from build123d import *

# Parameters (mm, degrees)
F0_R        = 19.05
F1_DEPTH    = 44.45
F2_W        = 88.9
F2_H        = 12.7
F3_DEPTH    = 44.45
F4_T1_DEPTH = 44.45
F5_R        = 9.525
F6_DEPTH    = 44.45
F7_W        = 50.8
F7_H        = 15.3564938247
F8_DEPTH    = 12.7
F9_R        = 7.62
F10_R       = 7.62
F11_R       = 9.525
F12_R       = 9.525


# Not quite as in the source:
# - a fillet or chamfer that OpenCascade refuses, or shapes differently, is made with other operations: its cross-section is extruded or revolved along the edge and cut away or added


with BuildPart() as f1:
    # F0 (on Front) → F1 (new body)
    with BuildSketch(Plane.XZ):
        with Locations((-59.2879876494, 38.2781662047)):
            Circle(F0_R)
    extrude(amount=F1_DEPTH)

    # F2 (on Front) → F3 (join)
    with BuildSketch(Plane.XZ):
        with Locations((-15.6031847, 49.8112538493)):
            Rectangle(F2_W, F2_H)
    extrude(amount=F3_DEPTH)

    # F4: fillet of radius 6.35 on 1 edges, made by hand

    # F4_s2 → F4_t1 (join)
    with BuildSketch(Plane.XZ):
        with BuildLine():
            add(Edge.make_bspline(
                [(-40.2581018773, 37.4029819382), (-39.9794820095, 43.4612538493), (-33.91480662, 43.4612538493)],
                knots=[0, 0, 0, 1, 1, 1], degree=2, weights=[1, 1, 1]))
            Line((-33.91480662, 43.4612538493), (-40.9566455691, 43.4612538493))
            ThreePointArc((-40.9566455691, 43.4612538493), (-40.3633740127, 40.4602520649), (-40.2581018773, 37.4029819382))
        make_face()
    extrude(amount=F4_T1_DEPTH)

    # F5 (on face) → F6 (cut)
    with BuildSketch(Plane.XZ.offset(44.45)):
        with Locations((-59.2879876494, 38.2781662047)):
            Circle(F5_R)
    extrude(amount=-F6_DEPTH, mode=Mode.SUBTRACT)

    # F7 (on face) → F8 (cut)
    with BuildSketch(Plane(origin=(0, 0, 43.4612538493), x_dir=(1, 0, 0), z_dir=(0, 0, -1))):
        with Locations((3.4468153, 21.9657469124)):
            Rectangle(F7_W, F7_H)
    extrude(amount=-F8_DEPTH, mode=Mode.SUBTRACT)

    # F9
    f9_edges = [f1.edges().sort_by_distance(p)[0] for p in [
        (-21.953185, -29.643994, 49.811254),
    ]]
    fillet(f9_edges, radius=F9_R)

    # F10
    f10_edges = [f1.edges().sort_by_distance(p)[0] for p in [
        (-21.953185, -14.2875, 49.811254),
    ]]
    fillet(f10_edges, radius=F10_R)

    # F11
    f11_edges = [f1.edges().sort_by_distance(p)[0] for p in [
        (28.846815, 0, 49.811254),
    ]]
    fillet(f11_edges, radius=F11_R)

    # F12
    f12_edges = [f1.edges().sort_by_distance(p)[0] for p in [
        (28.846815, -44.45, 49.811254),
    ]]
    fillet(f12_edges, radius=F12_R)


solid = f1.part
Verification items for the finished model (mm, model axes). A direction names the side the tool comes from. Give positions to 0.01 mm unless a question says otherwise; leave off trailing zeros. Loops run counter-clockwise (first coordinate to the right, second up) from the corner with the lowest first, then second, coordinate; pieces in that order, holes last.
1. Cross-section at B-B on z = 34. Record the cut outline in (x, y), and give its area (3 significant figures).
Derived:
outline: (-77.85, -44.45) - (-67.8, -44.45) - (-67.8, 0) - (-77.85, 0) - close; (-50.78, -44.45) - (-40.72, -44.45) - (-40.72, 0) - (-50.78, 0) - close
area: 894 mm2
2. Release check for a two-part mould opening along Y. For faces 6 (the cylindrical face through (25.983, -41.734, 49.9)), 7 (the cylindrical face through (26.131, -2.864, 49.9)), 8 (the cylindrical face through (-19.8, -16.6, 49.9)) record: +Y half, -Y half, draft (parallel to the pull), parting line (faces both ways), or undercut.
Derived:
face 6: -Y half
face 7: +Y half
face 8: undercut
3. Cross-section at A-A on x = 12.5. Record the cut outline in (y, z).
Derived:
outline: (-44.45, 43.46) - (-29.64, 43.46) - (-29.64, 56.16) - (-44.45, 56.16) - close; (-14.29, 43.46) - (0, 43.46) - (0, 56.16) - (-14.29, 56.16) - close
4. Cross-section at D-D on x = -32. Record the cut outline in (y, z), and give its area (3 significant figures).
Derived:
outline: (-44.45, 43.46) - (0, 43.46) - (0, 56.16) - (-44.45, 56.16) - close
area: 565 mm2
5. Material ranges on probe 1 along Y at (x, z) = (-0.5, 55.5); probe 2 along Z at (x, y) = (6.5, -13.5); probe 3 along Y at (x, z) = (-18, 45), recorded low to high.
Derived:
probe 1: y = -44.45 to -29.64, -14.29 to 0
probe 2: z = 43.46 to 56.16
probe 3: y = -44.45 to -28.7, -15.23 to 0
6. Tool access check on faces 1 (the flat face through (7, -29.644, 50)), 2 (the flat face through (28.847, -12, 50)), 3 (the cylindrical face through (-75.515, -21.914, 28.299)), 4 (the flat face through (-22, -27, 56.161)), 5 (the flat face through (-3, -12, 43.461)). Record the directions out of +Z, -Z, +X, -X, +Y, -Y that give a thin tool (end or side, any length) a straight path to the whole face; none if there is none.
Derived:
face 1: +Z, -Z, +X
face 2: +Z, -Z, +X, +Y, -Y
face 3: +Y, -Y
face 4: +Z, +X, +Y, -Y
face 5: -Z, +X, +Y, -Y
7. Go/stop test with flat-tipped pins: P1, Ø4, axis at y = -18, z = 42.5, coming from the -X side; P2, Ø4, axis at x = -22, y = -7, coming from the +Z side; P3, Ø5, axis at y = -20, z = 47.5, coming from the -X side. Record where each tip stops, or that it passes through.
Derived:
P1: stops at x = -78.21
P2: stops at z = 56.16
P3: stops at x = -77.11
